Geometry check sheet. Reference: the model listing, model coordinates, mm. A direction names the side the tool comes from. Round coordinates to 2 decimals unless told otherwise and drop trailing zeros. Loops run counter-clockwise (first coordinate to the right, second up) from the corner with the lowest first, then second, coordinate; pieces in that order, holes last.
Autodesk Inventor part; units mm, degrees
ref_plane "Start Plane" through (20, 0, 0) normal (1, 0, 0) x (0, 1, 0)
ref_plane "End Plane" through (150.5, 0, 0) normal (1, 0, 0) x (0, 1, 0)
ref_plane "XZ Plane" through (0, 0, 0) normal (0, 1, 0) x (-1, 0, 0)
ref_plane "Start Plane" through (20, 0, 0) normal (1, 0, 0) x (0, 1, 0)
ref_plane "End Plane" through (150.5, 0, 0) normal (1, 0, 0) x (0, 1, 0)
sketch "Sketch" plane through (0, 0, 0) normal (1, 0, 0) x (0, 1, 0)
  circle A0 centre (-3.0533, 11.4582) radius 2.1463
  line L0 (2.4543, 4.6976) -> (0.1995, 6.9525)
  arc A1 (1.8616, 3.2667) -> (2.4543, 4.6976) centre (1.8616, 4.1049) ccw
  line L1 (-0.2466, 3.2667) -> (1.8616, 3.2667)
  arc A2 (-0.2466, 3.2667) -> (-0.5514, 2.9619) centre (-0.2466, 2.9619) ccw
  line L2 (-0.5514, 2.2507) -> (-0.5514, 2.9619)
  arc A3 (-0.5514, 2.2507) -> (0.236, 1.4633) centre (0.236, 2.2507) ccw
  line L3 (4.935, 1.4633) -> (0.236, 1.4633)
  arc A4 (4.935, 1.4633) -> (6.9416, 3.4699) centre (4.935, 3.4699) ccw
  line L4 (6.9416, 8.1689) -> (6.9416, 3.4699)
  arc A5 (6.9416, 8.1689) -> (6.1542, 8.9563) centre (6.1542, 8.1689) ccw
  line L5 (5.443, 8.9563) -> (6.1542, 8.9563)
  arc A6 (5.443, 8.9563) -> (5.1382, 8.6515) centre (5.443, 8.6515) ccw
  line L6 (5.1382, 6.5433) -> (5.1382, 8.6515)
  arc A7 (3.7073, 5.9506) -> (5.1382, 6.5433) centre (4.3, 6.5433) ccw
  line L7 (1.4525, 8.2055) -> (3.7073, 5.9506)
  arc A8 (0.5746, 10.3248) -> (1.4525, 8.2055) centre (3.5718, 10.3248) ccw
  line L8 (0.5746, 12.5917) -> (0.5746, 10.3248)
  arc A9 (1.4525, 14.711) -> (0.5746, 12.5917) centre (3.5718, 12.5917) ccw
  line L9 (3.7073, 16.9658) -> (1.4525, 14.711)
  arc A10 (5.1382, 16.3731) -> (3.7073, 16.9658) centre (4.3, 16.3731) ccw
  line L10 (5.1382, 14.2649) -> (5.1382, 16.3731)
  arc A11 (5.1382, 14.2649) -> (5.443, 13.9601) centre (5.443, 14.2649) ccw
  line L11 (6.1542, 13.9601) -> (5.443, 13.9601)
  arc A12 (6.1542, 13.9601) -> (6.9416, 14.7475) centre (6.1542, 14.7475) ccw
  line L12 (6.9416, 19.4465) -> (6.9416, 14.7475)
  arc A13 (6.9416, 19.4465) -> (4.935, 21.4531) centre (4.935, 19.4465) ccw
  line L13 (0.236, 21.4531) -> (4.935, 21.4531)
  arc A14 (0.236, 21.4531) -> (-0.5514, 20.6657) centre (0.236, 20.6657) ccw
  line L14 (-0.5514, 19.9545) -> (-0.5514, 20.6657)
  arc A15 (-0.5514, 19.9545) -> (-0.2466, 19.6497) centre (-0.2466, 19.9545) ccw
  line L15 (1.8616, 19.6497) -> (-0.2466, 19.6497)
  arc A16 (2.4543, 18.2188) -> (1.8616, 19.6497) centre (1.8616, 18.8115) ccw
  line L16 (0.1995, 15.964) -> (2.4543, 18.2188)
  arc A17 (-1.9199, 15.0861) -> (0.1995, 15.964) centre (-1.9199, 18.0833) ccw
  line L17 (-4.1867, 15.0861) -> (-1.9199, 15.0861)
  arc A18 (-6.306, 15.964) -> (-4.1867, 15.0861) centre (-4.1867, 18.0833) ccw
  line L18 (-8.5609, 18.2188) -> (-6.306, 15.964)
  arc A19 (-7.9682, 19.6497) -> (-8.5609, 18.2188) centre (-7.9682, 18.8115) ccw
  line L19 (-5.86, 19.6497) -> (-7.9682, 19.6497)
  arc A20 (-5.86, 19.6497) -> (-5.5552, 19.9545) centre (-5.86, 19.9545) ccw
  line L20 (-5.5552, 20.6657) -> (-5.5552, 19.9545)
  arc A21 (-5.5552, 20.6657) -> (-6.3426, 21.4531) centre (-6.3426, 20.6657) ccw
  line L21 (-11.0416, 21.4531) -> (-6.3426, 21.4531)
  arc A22 (-11.0416, 21.4531) -> (-13.0482, 19.4465) centre (-11.0416, 19.4465) ccw
  line L22 (-13.0482, 14.7475) -> (-13.0482, 19.4465)
  arc A23 (-13.0482, 14.7475) -> (-12.2608, 13.9601) centre (-12.2608, 14.7475) ccw
  line L23 (-11.5496, 13.9601) -> (-12.2608, 13.9601)
  arc A24 (-11.5496, 13.9601) -> (-11.2448, 14.2649) centre (-11.5496, 14.2649) ccw
  line L24 (-11.2448, 16.3731) -> (-11.2448, 14.2649)
  arc A25 (-9.8139, 16.9658) -> (-11.2448, 16.3731) centre (-10.4066, 16.3731) ccw
  line L25 (-7.559, 14.711) -> (-9.8139, 16.9658)
  arc A26 (-6.6812, 12.5917) -> (-7.559, 14.711) centre (-9.6784, 12.5917) ccw
  line L26 (-6.6812, 10.3248) -> (-6.6812, 12.5917)
  arc A27 (-7.559, 8.2055) -> (-6.6812, 10.3248) centre (-9.6784, 10.3248) ccw
  line L27 (-9.8139, 5.9506) -> (-7.559, 8.2055)
  arc A28 (-11.2448, 6.5433) -> (-9.8139, 5.9506) centre (-10.4066, 6.5433) ccw
  line L28 (-11.2448, 8.6515) -> (-11.2448, 6.5433)
  arc A29 (-11.2448, 8.6515) -> (-11.5496, 8.9563) centre (-11.5496, 8.6515) ccw
  line L29 (-12.2608, 8.9563) -> (-11.5496, 8.9563)
  arc A30 (-12.2608, 8.9563) -> (-13.0482, 8.1689) centre (-12.2608, 8.1689) ccw
  line L30 (-13.0482, 3.4699) -> (-13.0482, 8.1689)
  arc A31 (-13.0482, 3.4699) -> (-11.0416, 1.4633) centre (-11.0416, 3.4699) ccw
  line L31 (-6.3426, 1.4633) -> (-11.0416, 1.4633)
  arc A32 (-6.3426, 1.4633) -> (-5.5552, 2.2507) centre (-6.3426, 2.2507) ccw
  line L32 (-5.5552, 2.9619) -> (-5.5552, 2.2507)
  arc A33 (-5.5552, 2.9619) -> (-5.86, 3.2667) centre (-5.86, 2.9619) ccw
  line L33 (-7.9682, 3.2667) -> (-5.86, 3.2667)
  arc A34 (-8.5609, 4.6976) -> (-7.9682, 3.2667) centre (-7.9682, 4.1049) ccw
  line L34 (-6.306, 6.9525) -> (-8.5609, 4.6976)
  arc A35 (-4.1867, 7.8303) -> (-6.306, 6.9525) centre (-4.1867, 4.8331) ccw
  line L35 (-1.9199, 7.8303) -> (-4.1867, 7.8303)
  arc A36 (0.1995, 6.9525) -> (-1.9199, 7.8303) centre (-1.9199, 4.8331) ccw
  point P0 (0, 0)
extrude "Body" add sketch "Sketch" along normal up to surface (130.5 mm away) from surface at 20
sketch "Sketch2" plane through (0, 0, 0) normal (1, 0, 0) x (0, 1, 0)
  line L0 (0, 0) -> (10, 0)
ref_plane "Work Plane3" through (0, 0, 0) normal (0, 0, -1) x (0, 1, 0)
sketch "Sketch3" plane through (0, 0, 0) normal (0, 0, -1) x (0, 1, 0)
  line L0 (-2, 20) -> (12, 20)
  line L1 (-2, 150.5) -> (12, 150.5)
  dimension "d7" = 130.5
equation "\"G_OFFSET_START\" = -20"
equation "\"G_OFFSET_END\" = -20"
equation "\"d2\" = -G_OFFSET_START"
equation "\"d3\" = length + G_OFFSET_END"
equation "\"G_L\" = d7"
properties part number "Generic-1"
1) Gauge pin test, flat ends, axial feed: pin 1 (0.6 mm diameter, centred on x = 117, y = -12, fed in from -Z); pin 2 (1.1 mm diameter, centred on x = 64.5, z = 12, fed in from -Y); pin 3 (0.6 mm diameter, centred on x = 99.5, y = -12, fed in from +Z). Record the tip position at first contact, or that the pin passes through.
Report:
pin 1: stops at z = 1.57
pin 2: stops at y = -6.68
pin 3: stops at z = 21.34
2) Sectioned sample at A-A, the plane y = -3. Record the cut outline in (x, z).
Report:
outline: (20, 7.83) - (150.5, 7.83) - (150.5, 9.31) - (20, 9.31) - close; (20, 13.6) - (150.5, 13.6) - (150.5, 15.09) - (20, 15.09) - close
3) Mould release check, pull along Y, two halves, no side actions. Record for faces 3 (the face through (84.34, -8.67, 15.82)), 4 (the face through (84.3, 6.4, 2.1)), 5 (the face through (84, -13.048, 17)), 6 (the face through (150.5, -5.4, 11.6)): +Y half, -Y half, draft (parallel to the pull), parting line (faces both ways), or undercut.
Report:
face 3: undercut
face 4: +Y half
face 5: -Y half
face 6: draft
4) Access from +Z, -Z, +X, -X, +Y, -Y to the whole of each face (thin tool, end or side, straight path). Record for faces 1 (the face through (84.34, -0.76, 15.32)), 2 (the face through (84, 3, 21.453)).
Report:
face 1: +X, -X
face 2: +Z, +X, -X, +Y, -Y
5) Scan lines: line 1 along Y through (x, z) = (51.5, 4); line 2 along Z through (x, y) = (144, -3.25); line 3 along Z through (x, y) = (61, 1.5). Record each from-to range of solid material in increasing order.
Report:
line 1: y = -13.05 to -8.8, 2.69 to 6.94
line 2: z = 7.83 to 9.32, 13.6 to 15.09
line 3: z = 1.46 to 3.27, 5.65 to 8.16, 14.76 to 17.26, 19.65 to 21.45
